Study the drawing (mm; zero at the part's minimum x, y, z) and answer. A direction names the side the tool comes from. Give positions to 0.01 mm unless a question says otherwise; leave off trailing zeros. Write each loop counter-clockwise with the first axis right and the second up, starting at its lowest first coordinate (ties: lowest second). Pieces come first, ordered by that corner, then holes. Notation, with made-up numbers: (-36, 15) -> (5, 15) arc R19 cw to (5, 37) -> close; hole circle Ø5 at (0, 46). An arc over 180 degrees is marked (long way). One line per question, with ' | ' between items.
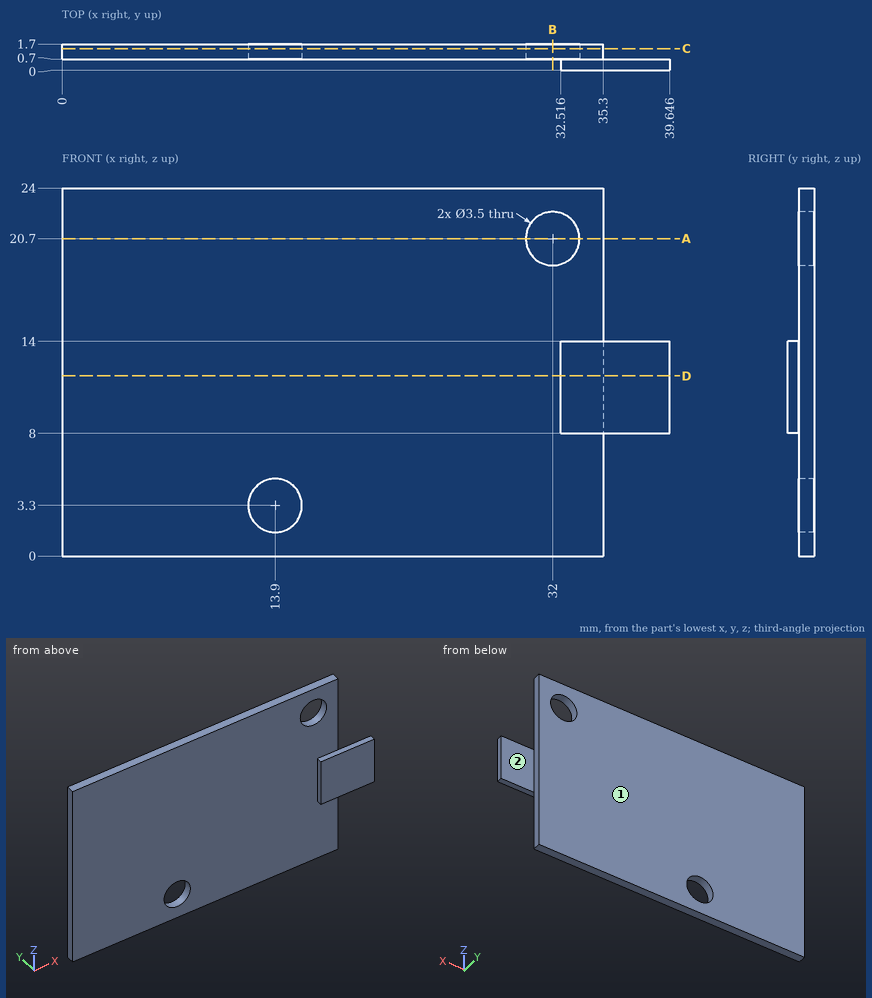
Item 1: Find section A-A (z = 20.7). Write down the section's boundary in (x, y).
Answers below:
outline: (0, 0.7) -> (30.25, 0.7) -> (30.25, 1.7) -> (0, 1.7) -> close; (33.75, 0.7) -> (35.3, 0.7) -> (35.3, 1.7) -> (33.75, 1.7) -> close
Item 2: Flat-ended cylindrical pins translate along their axes: pin 1 (0.8 mm diameter, centred on x = 35, y = 0.5, fed in from -Z); pin 2 (0.5 mm diameter, centred on y = 1, z = 14, fed in from +X); pin 3 (3 mm diameter, centred on x = 13.9, z = 3.3, fed in from -Y). Find the tip coordinate at first contact, or state that the pin passes through.
Answers below:
pin 1: z = 0 | pin 2: x = 35.3 | pin 3: through
Item 3: Find section D-D (z = 11.75). Write down the section's boundary in (x, y).
Answers below:
outline: (0, 0.7) -> (32.52, 0.7) -> (32.52, 0) -> (39.65, 0) -> (39.65, 0.7) -> (35.3, 0.7) -> (35.3, 1.7) -> (0, 1.7) -> close
Item 4: Find section C-C (y = 1.4). Write down the section's boundary in (x, z), then the cut area to 3 significant figures.
Answers below:
outline: (0, 0) -> (35.3, 0) -> (35.3, 24) -> (0, 24) -> close; hole circle Ø3.5 at (13.9, 3.3); hole circle Ø3.5 at (32, 20.7) | area: 828 mm²
Item 5: A tool of negligible diameter and unlimited length cuts with its end or side. For the marked faces 1 and 2, from which of +Z, -Z, +X, -X, +Y, -Y can it reach the whole face along a straight path? Write none if from no direction.
Answers below:
face 1: +Z, -Z, +X, -X, +Y | face 2: +Z, -Z, +X, +Y
Item 6: Find section B-B (x = 32). Write down the section's boundary in (y, z), then the cut area to 3 significant figures.
Answers below:
outline: (0.7, 0) -> (1.7, 0) -> (1.7, 18.95) -> (0.7, 18.95) -> close; (0.7, 22.45) -> (1.7, 22.45) -> (1.7, 24) -> (0.7, 24) -> close | area: 20.5 mm²
Item 7: Consider line 1 (Z direction, x = 13.9, y = 1); line 2 (Z direction, x = 32, y = 1.3); line 3 (Y direction, x = 34, z = 18.75). Determine where each line is inside the solid, lowest interval first. Write a range as [from, to].
Answers below:
line 1: [0, 1.55], [5.05, 24] | line 2: [0, 18.95], [22.45, 24] | line 3: [0.7, 1.7]
